Read the model definition and answer for the solid it produces. Units are mm, in the model's axes. Face numbers are marked on the shaded views. Round coordinates to 2 decimals unless told otherwise and drop trailing zeros. Loops run counter-clockwise (first coordinate to the right, second up) from the corner with the lowest first, then second, coordinate; pieces in that order, holes last. Notation, with made-up numbers: M 70.5,50 L 81.5,50 A13 cw 81.5,75 Z; hole C 33,-17 d2. An arc over 180 degrees is marked long. Write each question's results on one line, items separated by ' | '.
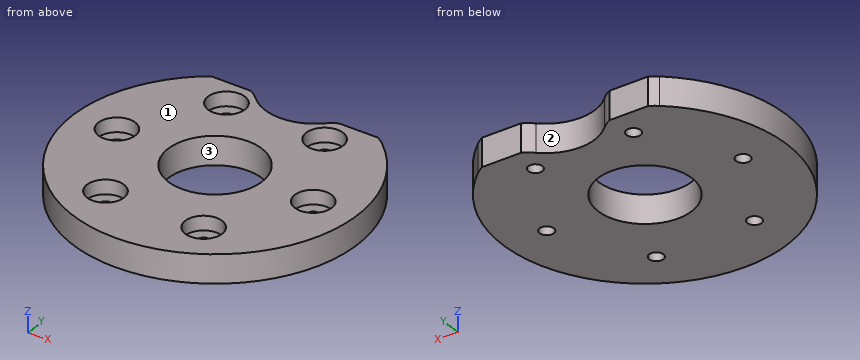
Autodesk Inventor part; units mm, degrees
ref_plane "YZ Plane" through (0, 0, 0) normal (1, 0, 0) x (0, 1, 0)
ref_plane "XZ Plane" through (0, 0, 0) normal (0, 1, 0) x (-1, 0, 0)
ref_plane "XY Plane" through (0, 0, 0) normal (0, 0, 1) x (1, 0, 0)
sketch "Sketch1" plane through (0, 0, 0) normal (0, 0, 1) x (1, 0, 0)
  circle A0 centre (0, 0) radius 50
  circle A1 centre (0, 0) radius 16.5
  circle A2 centre (35, 0) radius 2.5
  circle A3 centre (17.5, 30.3109) radius 2.5
  circle A4 centre (-17.5, 30.3109) radius 2.5
  circle A5 centre (-35, 0) radius 2.5
  circle A6 centre (-17.5, -30.3109) radius 2.5
  circle A7 centre (17.5, -30.3109) radius 2.5
  dimension "d0" = 100
  dimension "d1" = 33
  dimension "d2" = 5
  dimension "d3" = 35
  dimension "d6" = 360
extrude "Extrusion1" add sketch "Sketch1" along normal blind 10
sketch "Sketch2" plane through (0, 0, 10) normal (0, 0, 1) x (1, 0, 0)
  circle A0 centre (35, 0) radius 2.5
  circle A1 centre (35, 0) radius 6.5
  circle A2 centre (17.5, 30.3109) radius 6.5
  circle A3 centre (-17.5, 30.3109) radius 6.5
  circle A4 centre (-35, 0) radius 6.5
  circle A5 centre (-17.5, -30.3109) radius 6.5
  circle A6 centre (17.5, -30.3109) radius 6.5
  point P0 (0, 0)
  dimension "d10" = 13
  dimension "d13" = 360
extrude "Extrusion2" cut sketch "Sketch2" against normal blind 5 contours A0 | A1 | A2 | A3 | A4 | A5 | A6
sketch "Sketch3" plane through (0, 0, 10) normal (0, 0, 1) x (1, 0, 0)
  circle A0 centre (0, 0) radius 50 construction
  circle A1 centre (0, 50) radius 17.5
  dimension "d17" = 35
extrude "Extrusion3" cut sketch "Sketch3" against normal through all
fillet "Fillet1" radius 15 2 edges at (-17.2299, 46.9375, 5) (17.2299, 46.9375, 5)
sketch "Sketch4" plane through (0, 0, 10) normal (0, 0, 1) x (1, 0, 0)
  line L0 (-29.5557, 40.0005) -> (29.5557, 40.0005)
  arc A0 (-12.1932, 37.4471) -> (-32.3494, 38.125) centre (-22.6446, 26.6875) ccw construction
  arc A1 (32.3494, 38.125) -> (12.1932, 37.4471) centre (22.6446, 26.6875) ccw construction
  line L1 (-29.5557, 40.0005) -> (-29.5557, 42.0005)
  line L2 (-29.5557, 42.0005) -> (29.5557, 42.0005)
  line L3 (29.5557, 42.0005) -> (29.5557, 40.0005)
  point P0 (0, 0)
  dimension "d21" = 13.313
  dimension "d24" = 2
extrude "Extrusion4" cut sketch "Sketch4" against normal through all
properties part number "AA033" material "ABS Plastic"
Item 1: Flat-ended cylindrical pins translate along their axes: pin 1 (14.5 mm diameter, centred on x = 36, y = -2.5, fed in from +Z); pin 2 (3 mm diameter, centred on x = 17.5, y = 30.31, fed in from +Z); pin 3 (6.5 mm diameter, centred on x = 17.5, y = -30.31, fed in from +Z). Find the tip coordinate at first contact, or state that the pin passes through.
Outcome:
pin 1: stops at z = 10 | pin 2: passes through | pin 3: stops at z = 5
Item 2: Straight lines are drawn through the part: line 1 (Y direction, x = 18.5, z = 8); line 2 (Y direction, x = -17.5, z = 8.25); line 3 (X direction, y = 29.5, z = 0.75). For each, find the intervals that lie inside material, in ascending order.
Outcome:
line 1: y = -46.45 to -36.73, -23.89 to 23.89, 36.73 to 40 | line 2: y = -46.84 to -36.81, -23.81 to 23.81, 36.81 to 40 | line 3: x = -40.37 to -19.86, -15.14 to 15.14, 19.86 to 40.37
Item 3: The part is cut by section B-B (x = 35). Determine the outline of the cut face in (y, z).
Outcome:
outline: M -35.71,0 L -2.5,0 L -2.5,5 L -6.5,5 L -6.5,10 L -35.71,10 Z; M 2.5,0 L 35.71,0 L 35.71,10 L 6.5,10 L 6.5,5 L 2.5,5 Z
Item 4: The mould has two halves that part along Y. Classify the marked faces 1, 2 and 3: pulls with the +Y half, pulls with the -Y half, needs draft (parallel to the pull), parting line crosses it, or undercut.
Outcome:
face 1: needs draft | face 2: pulls with the +Y half | face 3: undercut
Item 5: The part is cut by section A-A (y = 0). Determine the outline of the cut face in (x, z), plus the area to 3 significant figures.
Outcome:
outline: M -50,0 L -37.5,0 L -37.5,5 L -41.5,5 L -41.5,10 L -50,10 Z; M -32.5,0 L -16.5,0 L -16.5,10 L -28.5,10 L -28.5,5 L -32.5,5 Z; M 16.5,0 L 32.5,0 L 32.5,5 L 28.5,5 L 28.5,10 L 16.5,10 Z; M 37.5,0 L 50,0 L 50,10 L 41.5,10 L 41.5,5 L 37.5,5 Z | area: 490 mm2
Item 6: The part is cut by section D-D (z = 3.5). State how many separate pieces and enclosed holes the cut face has, plus the area to 3 significant figures.
Outcome:
separate pieces: 1 | enclosed holes: 7 | area: 6,320 mm2
Item 7: The part is cut by section C-C (y = 14). Determine the outline of the cut face in (x, z).
Outcome:
outline: M -48,0 L -8.73,0 L -8.73,10 L -48,10 Z; M 8.73,0 L 48,0 L 48,10 L 8.73,10 Z
